Input: dimensioned drawing with shaded views. Units: mm. Origin: part minimum x, y, z. A direction names the side the tool comes from. Give positions to 0.01 mm unless a question says otherwise; leave off trailing zeros. Order: outer loops, then holes, each group sorted by start corner. A loop starts at its lowest first (then second) coordinate and runs counter-clockwise, first axis right, second up. Notation, with made-up numbers: (78, 24) -> (91, 24) arc R18 cw to (91, 48) -> close; hole circle Ø6 at (-5, 27.5). An arc over 180 degrees is marked (long way). One line per question, with ' | ' between items. Start each with the question number.
(1) Section A-A (x = 2). Return loops of the section in (y, z).
(2) Section C-C (z = 8). Return loops of the section in (x, y), then the cut area to 3 significant figures.
(3) Section B-B (y = 28). Return loops of the section in (x, z).
(4) Set-up query: the marked faces 1, 2 and 3. Return all of +Z, -Z, +X, -X, +Y, -Y with unobstructed straight access to the full face (end or side cutting, diameter ignored); none if empty.
(5) First-contact query: pin 1 Ø10 at (x, z) = (6, 6.5) entering from +Y; pin 2 Ø2 at (x, y) = (15.5, 58.5) entering from -Z; pin 3 Ø4 at (y, z) = (29.5, 39) entering from -X; pin 4 Ø10 at (x, y) = (10.5, 56.5) entering from +Z. Flat tips, straight axial feed; report the tip coordinate or a pass-through.
(6) Ray query, L1, parallel to Z at x = 2.75, y = 66.5; L2, parallel to Y at x = 5.75, z = 114. Return the intervals inside material, ascending.
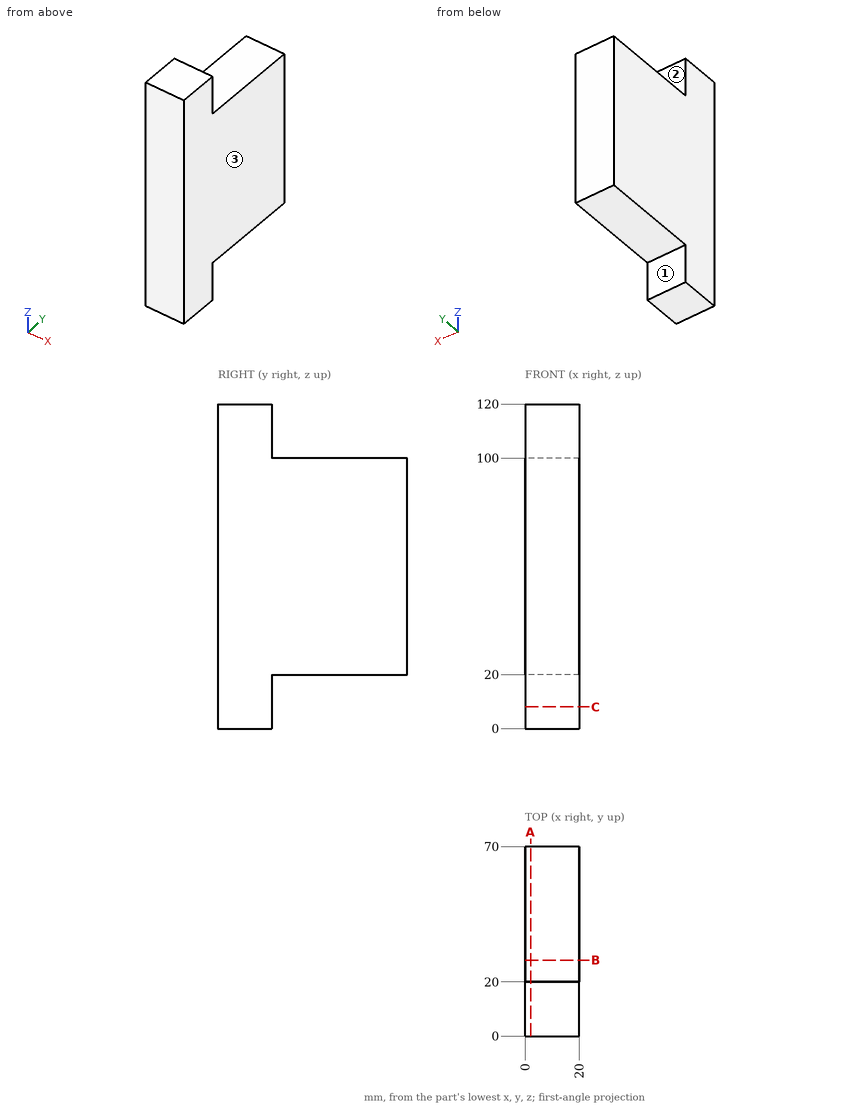
Response:
1) outline: (0, 0) -> (20, 0) -> (20, 20) -> (70, 20) -> (70, 100) -> (20, 100) -> (20, 120) -> (0, 120) -> close
2) outline: (0, 0) -> (20, 0) -> (20, 20) -> (0, 20) -> close | area: 400 mm^2
3) outline: (0, 20) -> (20, 20) -> (20, 100) -> (0, 100) -> close
4) face 1: -Z, +X, -X, +Y | face 2: +Z, +X, -X, +Y | face 3: +Z, -Z, +X, +Y, -Y
5) pin 1: stops at y = 20 | pin 2: stops at z = 20 | pin 3: stops at x = 0 | pin 4: stops at z = 100
6) L1: z = 20 to 100 | L2: y = 0 to 20
